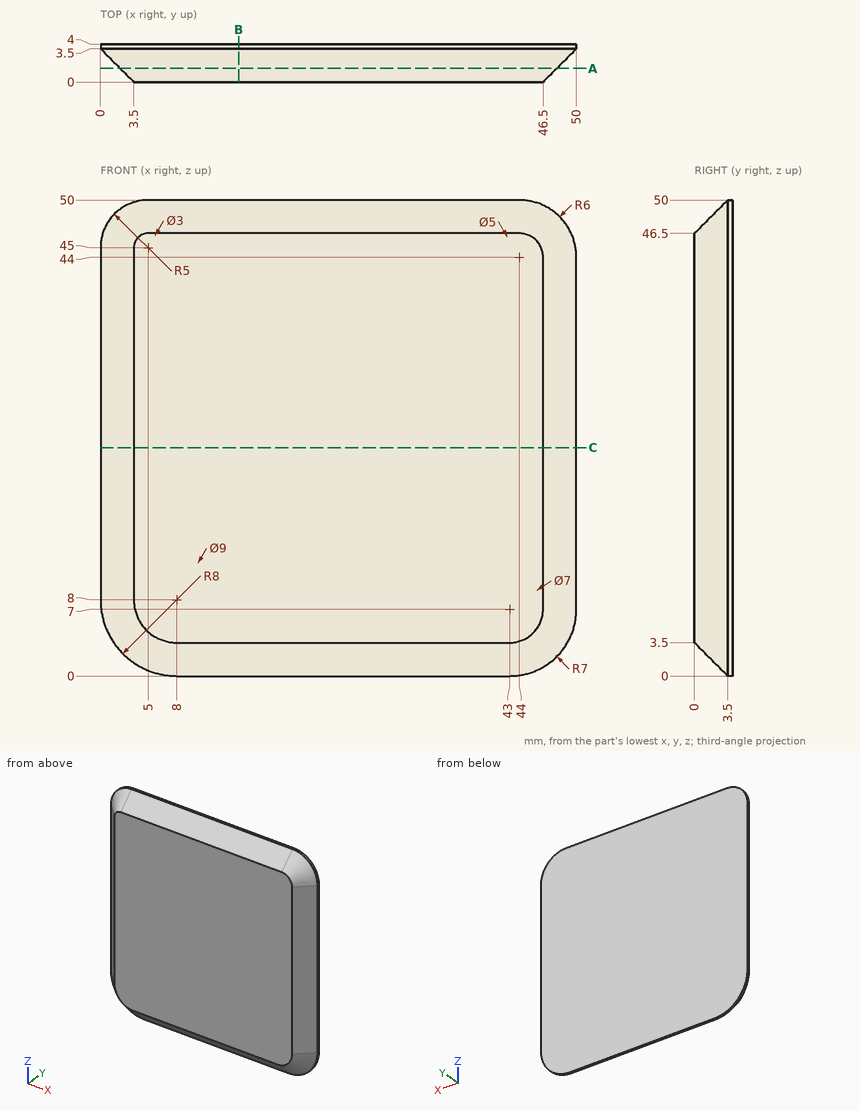
Geometry check sheet. Reference: drawing and pictorial views, mm from the part's lowest x, y, z. Give positions to 0.01 mm unless a question says otherwise; leave off trailing zeros. Loops run counter-clockwise (first coordinate to the right, second up) from the corner with the lowest first, then second, coordinate; pieces in that order, holes last. Notation, with made-up numbers: M 34,78 L 44,78 A17 cw 44,83 Z; hole C 73,45 d4. An arc over 180 degrees is marked long. Use a Markdown table: item, result. Add a question column.
Q1. Sectioned sample at B-B, the plane x = 14.5. Record the cut outline in (y, z), then the cut area to 3 significant figures.
Q2. Sectioned sample at C-C, the plane z = 24. Record the cut outline in (x, y).
Q3. Scan lines: line 1 along Z through (x, y) = (20, 1.75); line 2 along Z through (x, y) = (9.5, 2.2); line 3 along X through (y, z) = (0.4, 31). Record each from-to range of solid material in increasing order. Write a range as [from, to].
Q4. Go/stop test with flat-tipped pins: pin 1 (1 mm diameter, centred on x = 39.5, y = 1.5, fed in from -Z); pin 2 (2 mm diameter, centred on y = 1, z = 9, fed in from -X). Record where each tip stops, or that it passes through.
Q5. Sectioned sample at A-A, the plane y = 1.45. Record the cut outline in (x, z), then the cut area to 3 significant figures.
Verdict:
| question | item | result |
|---|---|---|
| 1 | outline | M 0,3.5 L 3.5,0 L 4,0 L 4,50 L 3.5,50 L 0,46.5 Z |
| 1 | area | 188 mm^2 |
| 2 | outline | M 0,3.5 L 3.5,0 L 46.5,0 L 50,3.5 L 50,4 L 0,4 Z |
| 3 | line 1 | [1.75, 48.25] |
| 3 | line 2 | [1.3, 48.7] |
| 3 | line 3 | [3.1, 46.9] |
| 4 | pin 1 | z = 1.5 |
| 4 | pin 2 | x = 1.5 |
| 5 | outline | M 2.05,8 A5.95 ccw 8,2.05 L 43,2.05 A4.95 ccw 47.95,7 L 47.95,44 A3.95 ccw 44,47.95 L 5,47.95 A2.95 ccw 2.05,45 Z |
| 5 | area | 2,090 mm^2 |
